Source: CAD feature listing. Evaluate the final solid. Frame: model axes, mm. Coordinates: 2 decimals unless noted, no trailing zeros. Order: outer loops, then holes, each group sorted by start corner. A loop starts at its lowest first (then second) coordinate and runs counter-clockwise, first axis right, second up. Notation, with made-up numbers: (-15.5, -27.5) -> (9.5, -27.5) arc R20 ccw to (9.5, -21.5) -> close; hole circle Ø5 at (-4.75, -36.75). An arc over 180 degrees is marked (long way). Put each result on its own line as item: value.
from build123d import *

# Parameters (mm, degrees)
BOSS_EXTRUDE1_DEPTH         = 9.525
F_3_8_CLEARANCE_HOLE1_D     = 10.0838
F_3_8_CLEARANCE_HOLE1_DEPTH = 25.4
F_3_8_CLEARANCE_HOLE1_TIP   = 3.029479155


with BuildPart() as part:
    # Sketch1 → Boss-Extrude1 (new body)
    with BuildSketch(Plane.XY):
        Polygon((-228.6, -36.83), (-228.6, -189.23), (228.6, -189.23), (228.6, -36.83), (228.6, 191.77), (-228.6, 191.77), align=None)
    extrude(amount=BOSS_EXTRUDE1_DEPTH)

    # 3/8 Clearance Hole1
    with Locations(Plane.XY.offset(9.525)):
        with Locations((-215.9, 179.07), (215.9, 179.07), (196.85, -176.53), (-196.85, -176.53)):
            Hole(F_3_8_CLEARANCE_HOLE1_D / 2, depth=F_3_8_CLEARANCE_HOLE1_DEPTH)
            with Locations((0, 0, -(F_3_8_CLEARANCE_HOLE1_DEPTH + F_3_8_CLEARANCE_HOLE1_TIP / 2))):  # 118° drill point
                Cone(0, F_3_8_CLEARANCE_HOLE1_D / 2, F_3_8_CLEARANCE_HOLE1_TIP, mode=Mode.SUBTRACT)


solid = part.part
1. Cut plane A-A on y = 179.07. Output: boundary loops of the cut face in (x, z) (3 decimals), plus the area to 3 significant figures.
Numbers:
outline: (-228.6, 0) -> (-220.942, 0) -> (-220.942, 9.525) -> (-228.6, 9.525) -> close; (-210.858, 0) -> (210.858, 0) -> (210.858, 9.525) -> (-210.858, 9.525) -> close; (220.942, 0) -> (228.6, 0) -> (228.6, 9.525) -> (220.942, 9.525) -> close
area: 4,160 mm2
2. Ray query, line 1 along Y through (x, z) = (196.85, 7.5); line 2 along Y through (x, z) = (-215.9, 6.75). Return the intervals inside material, ascending.
Numbers:
line 1: y = -189.23 to -181.57, -171.49 to 191.77
line 2: y = -189.23 to 174.03, 184.11 to 191.77
3. Pull-direction query (X, two-part tool) for faces 1 (the cylindrical face through (220.937, 179.292, 4.696)), 2 (the flat face through (-228.6, 4, 5)), 3 (the flat face through (-3, 4, 0)); classes: pulls with the +X half, pulls with the -X half, needs draft (parallel to the pull), parting line crosses it, or undercut.
Numbers:
face 1: undercut
face 2: pulls with the -X half
face 3: needs draft
4. First-contact query: pin 1 (6 mm diameter, centred on x = 5.5, y = 22.5, fed in from -Z). Flat tip, straight axial feed; report the tip coordinate or a pass-through.
Numbers:
pin 1: stops at z = 0
5. Cut plane B-B on x = 196.85. Output: boundary loops of the cut face in (y, z) (3 decimals), plus the area to 3 significant figures.
Numbers:
outline: (-189.23, 0) -> (-181.572, 0) -> (-181.572, 9.525) -> (-189.23, 9.525) -> close; (-171.488, 0) -> (191.77, 0) -> (191.77, 9.525) -> (-171.488, 9.525) -> close
area: 3,530 mm2
